Read the model definition and answer for the solid it produces. Units are mm, in the model's axes. Face numbers are marked on the shaded views. A direction names the side the tool comes from. Coordinates: 2 decimals unless noted, no trailing zeros. Loops run counter-clockwise (first coordinate to the right, second up) from the corner with the lowest first, then second, coordinate; pieces in that order, holes last. Notation, with made-up numbers: (-31.5, -31) -> (-10.5, -31) arc R7 ccw to (-10.5, -19) -> close; hole circle Ø3 at (-19.5, 70.5). An arc over 180 degrees is marked (long way). Answer as a JSON object with one key per item and string values. Group by question number.
Q1. The part is cut by section D-D on y = -34. Write down the section's boundary in (x, z), and give its area (3 significant figures).
Q2. The part is cut by section B-B on x = -19. Write down the section's boundary in (y, z), and give its area (3 significant figures).
Q3. Each of these flat-tipped pins is pushed along its axis until it touches: P1, Ø4, axis at y = 39.5, z = 19, coming from the +X side; P2, Ø4, axis at x = -15.5, z = 16.5, coming from the +Y side; P3, Ø4, axis at y = 21, z = 9.5, coming from the +X side; P4, Ø2.5, axis at y = 40.5, z = 14.5, coming from the -X side. Where does it stop, or does it pass through?
Q4. The part is cut by section A-A on y = 0. Write down the section's boundary in (x, z), and give its area (3 significant figures).
Q5. Determine the mould class of the marked faces 1, 2, 3 and 4 for opening direction X: released by +X, released by -X, zero draft, split by the parting line, or undercut.
Q6. Straight lines are drawn through the part: line 1 along Y through (x, z) = (-1, 4.5); line 2 along Z through (x, y) = (-27, 14); line 3 along X through (y, z) = (21, 3.75). For each, find the intervals that lie inside material, in ascending order. Write a range as [from, to].
Q7. For the marked faces 5 and 6, determine the directions among +Z, -Z, +X, -X, +Y, -Y from which every point of the face is accessible in a straight line to the end or side of a thin tool.
Q8. The part is cut by section C-C on z = 22.5. Write down the section's boundary in (x, y).
from build123d import *

# Parameters (mm, degrees)
F0_R         = 37
F0_R_2       = 35.5
F1_DEPTH     = 30
F2_W         = 100
F2_H         = 30
F3_DEPTH     = 15
F6_R         = 35.5
F6_R_2       = 29
F7_DEPTH     = 15
F8_W         = 5
F8_H         = 5
F9_DEPTH     = 25
F10_T4_DEPTH = 108.868862808
F10_S5_R     = 37
F10_T6_DEPTH = 57
F11_W        = 5
F11_H        = 5
F12_DEPTH    = 25
F13_T4_DEPTH = 108.868862808
F13_S5_R     = 37
F13_T6_DEPTH = 57


# Not quite as in the source:
# - a fillet or chamfer that OpenCascade refuses, or shapes differently, is made with other operations: its cross-section is extruded or revolved along the edge and cut away or added


with BuildPart() as f1:
    # F0 (on Top) → F1 (new body)
    with BuildSketch(Plane.XY):
        Circle(F0_R)
        Circle(F0_R_2, mode=Mode.SUBTRACT)
    extrude(amount=F1_DEPTH)


with BuildPart() as f3:
    # F2 (on Top) → F3 (new body)
    with BuildSketch(Plane.XY):
        Rectangle(F2_W, F2_H)
    extrude(amount=F3_DEPTH)


with BuildPart() as f3_1:
    # F4: moved
    add(f3.part.moved(Location((0, 0, 15))))


with BuildPart() as f1_1:
    add(f1.part)

    # F5: cut F3
    add(f3_1.part, mode=Mode.SUBTRACT)

    # F6 (on Top) → F7 (join)
    with BuildSketch(Plane.XY):
        Circle(F6_R)
        Circle(F6_R_2, mode=Mode.SUBTRACT)
    extrude(amount=F7_DEPTH)

    # F8 (on face) → F9 (join)
    with BuildSketch(Plane.XY.offset(30)):
        with Locations((0, -39.4154439226)):
            Rectangle(F8_W, F8_H)
    extrude(amount=-F9_DEPTH)

    # F10: chamfer of 20 x 5.3589838486 on 1 edges, made by hand


with BuildPart() as f10_tool2:
    # F10_s3 → F10_t4 (new body)
    with BuildSketch(Plane.YZ.offset(-54.434431404)):
        Polygon((-36.5564600739, 5), (-41.9154439226, 25), (-41.9154439226, 5), align=None)
    extrude(amount=F10_T4_DEPTH)

    # F10_s5 → F10_t6 (cut, symmetric)
    with BuildSketch(Plane.XY.offset(15)):
        Circle(F10_S5_R)
    extrude(amount=F10_T6_DEPTH, both=True, mode=Mode.SUBTRACT)


with BuildPart() as f1_2:
    add(f1_1.part)

    # F10_t1: cut F10_tool2
    add(f10_tool2.part, mode=Mode.SUBTRACT)

    # F11 (on face) → F12 (join)
    with BuildSketch(Plane.XY.offset(30)):
        with Locations((0, 39.3967875838)):
            Rectangle(F11_W, F11_H)
    extrude(amount=-F12_DEPTH)

    # F13: chamfer of 20 x 5.3589838486 on 1 edges, made by hand


with BuildPart() as f13_tool2:
    # F13_s3 → F13_t4 (new body)
    with BuildSketch(Plane.YZ.offset(54.434431404)):
        Polygon((36.5378037352, 5), (41.8967875838, 25), (41.8967875838, 5), align=None)
    extrude(amount=-F13_T4_DEPTH)

    # F13_s5 → F13_t6 (cut, symmetric)
    with BuildSketch(Plane.XY.offset(15)):
        Circle(F13_S5_R)
    extrude(amount=F13_T6_DEPTH, both=True, mode=Mode.SUBTRACT)


with BuildPart() as f1_3:
    add(f1_2.part)

    # F13_t1: cut F13_tool2
    add(f13_tool2.part, mode=Mode.SUBTRACT)


solid = f1_3.part
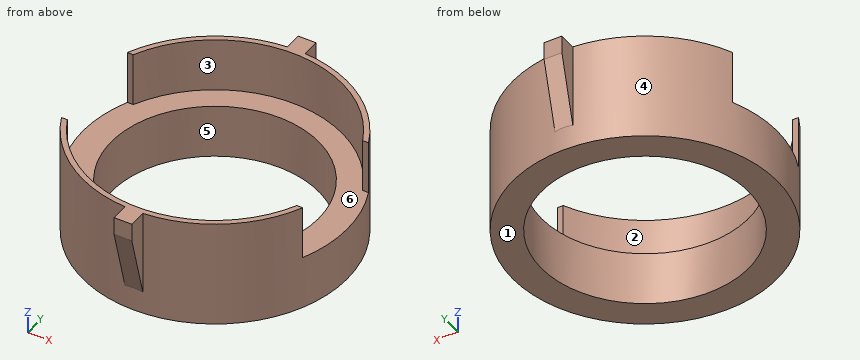
Final values:
{
 "1": {"outline": "(-14.59, 0) -> (14.59, 0) -> (14.59, 30) -> (10.21, 30) -> (10.21, 15) -> (-10.21, 15) -> (-10.21, 30) -> (-14.59, 30) -> close", "area": "569 mm2"},
 "2": {"outline": "(-31.75, 0) -> (-21.91, 0) -> (-21.91, 15) -> (-29.99, 15) -> (-29.99, 30) -> (-31.75, 30) -> close; (21.91, 0) -> (31.75, 0) -> (31.75, 30) -> (29.99, 30) -> (29.99, 15) -> (21.91, 15) -> close", "area": "348 mm2"},
 "3": {"P1": "stops at x = 2.5", "P2": "stops at y = 34.45", "P3": "stops at x = 31.75", "P4": "passes through"},
 "4": {"outline": "(-37, 0) -> (-29, 0) -> (-29, 15) -> (-37, 15) -> close; (29, 0) -> (37, 0) -> (37, 15) -> (29, 15) -> close", "area": "240 mm2"},
 "5": {"face 1": "zero draft", "face 2": "undercut", "face 3": "undercut", "face 4": "split by the parting line"},
 "6": {"line 1": "y = [-36.99, -28.98], [28.98, 36.99]", "line 2": "z = [0, 15]", "line 3": "x = [-30.46, -20], [20, 30.46]"},
 "7": {"face 5": "+Z, -Z", "face 6": "+Z"},
 "8": {"outline": "(-33.82, -15) arc R37 ccw to (-2.5, -36.92) -> (-2.5, -41.25) -> (2.5, -41.25) -> (2.5, -36.92) arc R37 ccw to (33.82, -15) -> (32.18, -15) arc R35.5 cw to (-32.18, -15) -> close; (-33.82, 15) -> (-32.18, 15) arc R35.5 cw to (32.18, 15) -> (33.82, 15) arc R37 ccw to (2.5, 36.92) -> (2.5, 41.23) -> (-2.5, 41.23) -> (-2.5, 36.92) arc R37 ccw to start"}
}
